Verification items for this drawing (mm, ordinates from the low corner). A direction names the side the tool comes from. Round coordinates to 2 decimals unless told otherwise and drop trailing zeros. Order: outer loops, then holes, each group sorted by start corner. A loop starts at its lowest first (then second) coordinate and runs counter-clockwise, first axis right, second up. Notation, with made-up numbers: (-6.75, 60.25) -> (-1.75, 60.25) arc R11 ccw to (-1.75, 80.25) -> close; hole circle Ø10 at (41, -20). An arc over 180 degrees is marked (long way). Return JSON: item names as keys, results as strings. Group by question number.
Item 1: Sectioned sample at C-C on x = 29. Record the cut outline in (y, z), plus the area to 3 significant figures.
Item 2: Scan lines: probe 1 along Y at (x, z) = (30, 30); probe 2 along Z at (x, y) = (3, 3.25); probe 3 along Z at (x, y) = (36, 8.5). Record each from-to range of solid material in increasing order. Write a range as from..to.
Item 3: Sectioned sample at B-B on z = 9. Record the cut outline in (x, y), plus the area to 3 significant figures.
Item 4: Sectioned sample at D-D on z = 15. Record the cut outline in (x, y).
Item 5: Access from +Z, -Z, +X, -X, +Y, -Y to the whole of each face (thin tool, end or side, straight path). Record for the marked faces 1 and 2.
Item 6: Depth check by flat-ended pin: pin 1 Ø13 at (x, z) = (26.5, 23.5) entering from -Y; pin 2 Ø5 at (x, y) = (42.5, 10) entering from +Z; pin 3 Ø2 at (y, z) = (11.5, 25.5) entering from +X; pin 4 Ø5 at (x, y) = (26.5, 10) entering from -Z. Enter the tip coordinate at first touch or a pass-through.
Item 7: Sectioned sample at A-A on x = 12.5. Record the cut outline in (y, z), plus the area to 3 significant figures.
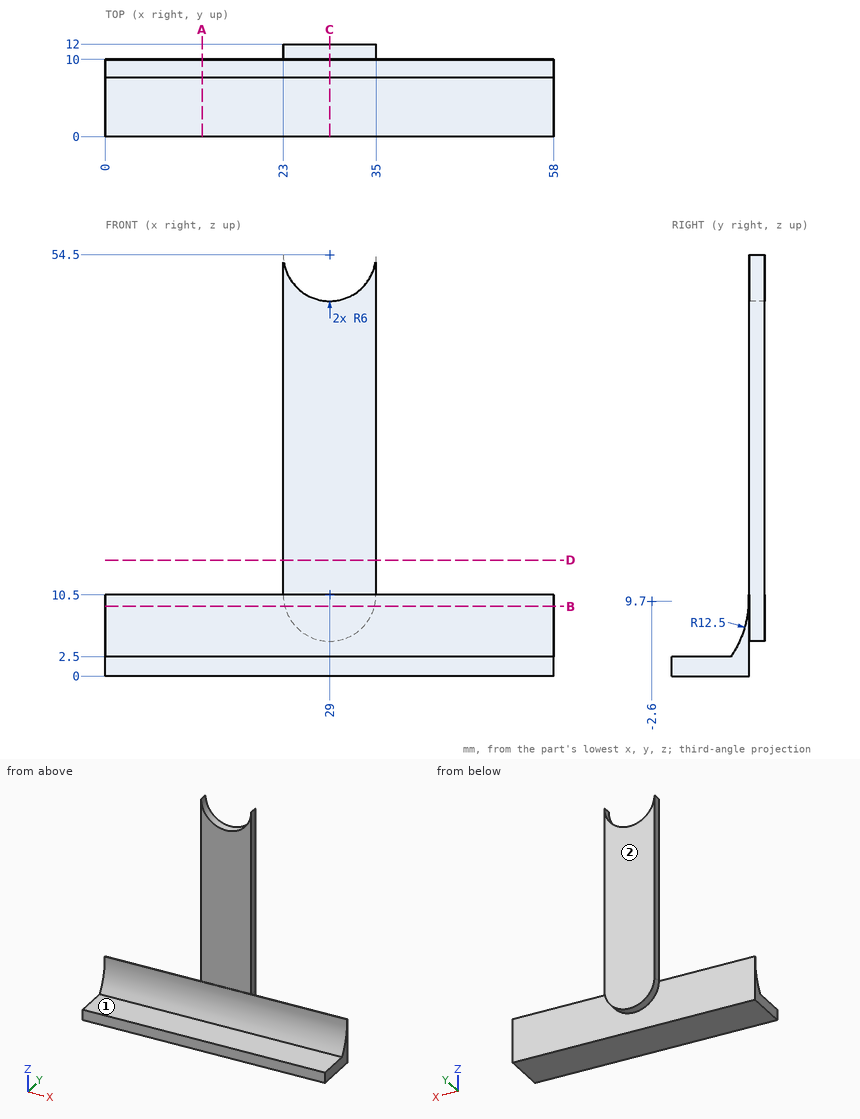
Recorded:
{
 "1": {"outline": "(0, 0) -> (10, 0) -> (10, 4.5) -> (12, 4.5) -> (12, 48.5) -> (10, 48.5) -> (10, 10.5) -> (9.87, 10.5) arc R12.5 cw to (7.62, 2.5) -> (0, 2.5) -> close", "area": "119 mm²"},
 "2": {"probe 1": "10..12", "probe 2": "0..2.5", "probe 3": "0..3.95"},
 "3": {"outline": "(0, 9.88) -> (58, 9.88) -> (58, 10) -> (34.81, 10) -> (34.81, 12) -> (23.19, 12) -> (23.19, 10) -> (0, 10) -> close", "area": "30.2 mm²"},
 "4": {"outline": "(23, 10) -> (35, 10) -> (35, 12) -> (23, 12) -> close"},
 "5": {"face 1": "+Z, +X, -X, -Y", "face 2": "+Z, -Z, +X, -X, +Y"},
 "6": {"pin 1": "y = 10", "pin 2": "z = 10.5", "pin 3": "x = 35", "pin 4": "z = 0"},
 "7": {"outline": "(0, 0) -> (10, 0) -> (10, 10.5) -> (9.87, 10.5) arc R12.5 cw to (7.62, 2.5) -> (0, 2.5) -> close", "area": "31.1 mm²"}
}
